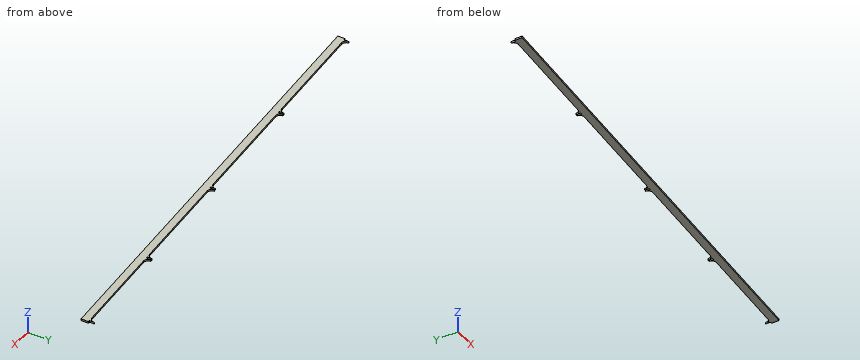
from build123d import *

# Parameters (mm, degrees)
EXTRUDE_1_DEPTH = 2


with BuildPart() as part:
    # 草图1 → 凸台-拉伸1 (new body)
    with BuildSketch(Plane.XY):
        with BuildLine():
            Line((5.593665372, 13.939609945), (3.593665372, 13.939609945))
            Line((3.593665372, 13.939609945), (3.593665372, 5.539609945))
            Line((3.593665372, 5.539609945), (528.593665372, 41.925528217))
            Line((528.593665372, 41.925528217), (528.593665372, 50.186915195))
            Line((528.593665372, 50.186915195), (526.593665372, 50.186915195))
            Line((526.593665372, 50.186915195), (526.593665372, 55.785469044))
            ThreePointArc((526.593665372, 55.785469044), (524.980524361, 51.692124664), (521.008509302, 49.799827515))
            Line((521.008509302, 49.799827515), (415.939368647, 42.517851963))
            ThreePointArc((415.939368647, 42.517851963), (412.182545056, 43.850170746), (410.593665372, 47.50588657))
            Line((410.593665372, 47.50588657), (410.593665372, 42.008746898))
            Line((410.593665372, 42.008746898), (408.593665372, 42.008746898))
            Line((408.593665372, 42.008746898), (408.593665372, 47.607300746))
            ThreePointArc((408.593665372, 47.607300746), (406.980524361, 43.513956367), (403.008509302, 41.621659217))
            Line((403.008509302, 41.621659217), (285.939368647, 33.508005533))
            ThreePointArc((285.939368647, 33.508005533), (282.182545056, 34.840324317), (280.593665372, 38.496040141))
            Line((280.593665372, 38.496040141), (280.593665372, 32.998900469))
            Line((280.593665372, 32.998900469), (278.593665372, 32.998900469))
            Line((278.593665372, 32.998900469), (278.593665372, 38.597454317))
            ThreePointArc((278.593665372, 38.597454317), (276.980524361, 34.504109938), (273.008509302, 32.611812788))
            Line((273.008509302, 32.611812788), (145.939368647, 23.805093994))
            ThreePointArc((145.939368647, 23.805093994), (142.182545056, 25.137412778), (140.593665372, 28.793128602))
            Line((140.593665372, 28.793128602), (140.593665372, 23.29598893))
            Line((140.593665372, 23.29598893), (138.593665372, 23.29598893))
            Line((138.593665372, 23.29598893), (138.593665372, 28.894542778))
            ThreePointArc((138.593665372, 28.894542778), (136.980524361, 24.801198399), (133.008509302, 22.908901249))
            Line((133.008509302, 22.908901249), (10.939368647, 14.44871501))
            ThreePointArc((10.939368647, 14.44871501), (7.182545056, 15.781033793), (5.593665372, 19.436749618))
            Line((5.593665372, 19.436749618), (5.593665372, 13.939609945))
        make_face()
    extrude(amount=EXTRUDE_1_DEPTH)


solid = part.part
Build history of the part. All positions in model axes, mm. Round coordinates to 2 decimals unless told otherwise and drop trailing zeros. Write each loop counter-clockwise with the first axis right and the second up, starting at its lowest first coordinate (ties: lowest second). Pieces come first, ordered by that corner, then holes. Notation, with made-up numbers: M 8,38.5 L 63,38.5 A36 ccw 63,74.5 Z; hole C 72,0.5 d11. An arc over 180 degrees is marked long. Use CSV: the item, a comma, the result in double quotes.
1. Wall check: probe 1 along Y at (x, z) = (493.5, 0.9); probe 2 along Y at (x, z) = (154, 0.5); probe 3 along X at (y, z) = (52, 1.3). Give the ranges that are in metal, low to high. Write a range as from..to.
Reply:
probe 1,"y = 39.49..47.89"
probe 2,"y = 15.96..24.36"
probe 3,"x = 525.25..526.59"
2. Saw through at A-A (z = 0.65). Give the cut face in (x, y), plus the area to 3 significant figures.
Reply:
outline,"M 3.59,5.54 L 528.59,41.93 L 528.59,50.19 L 526.59,50.19 L 526.59,55.79 A6 cw 521.01,49.8 L 415.94,42.52 A5 cw 410.59,47.51 L 410.59,42.01 L 408.59,42.01 L 408.59,47.61 A6 cw 403.01,41.62 L 285.94,33.51 A5 cw 280.59,38.5 L 280.59,33 L 278.59,33 L 278.59,38.6 A6 cw 273.01,32.61 L 145.94,23.81 A5 cw 140.59,28.79 L 140.59,23.3 L 138.59,23.3 L 138.59,28.89 A6 cw 133.01,22.91 L 10.94,14.45 A5 cw 5.59,19.44 L 5.59,13.94 L 3.59,13.94 Z"
area,"4,460 mm²"
3. Saw through at B-B (x = 56). Give the cut face in (y, z).
Reply:
outline,"M 9.17,0 L 17.57,0 L 17.57,2 L 9.17,2 Z"
4. Flat gauge pins, fed straight in: pin 1 (1 mm diameter, centred on x = 4, z = 1, fed in from +Y); pin 2 (1 mm diameter, centred on y = 35.5, z = 1.5, fed in from -X); pin 3 (0.6 mm diameter, centred on y = 18, z = 1, fed in from -X); pin 4 (3 mm diameter, centred on x = 178, y = 23.5, fed in from -Z). Where does each tip first touch, or does it go through?
Reply:
pin 1,"stops at y = 13.94"
pin 2,"stops at x = 277.4"
pin 3,"stops at x = 5.59"
pin 4,"stops at z = 0"
